Work out the finished part from the listing and answer in its coordinate system (mm). Face numbers are marked on the shaded views. A direction names the side the tool comes from. Coordinates: 2 decimals unless noted, no trailing zeros. Loops run counter-clockwise (first coordinate to the right, second up) from the corner with the lowest first, then second, coordinate; pieces in that order, holes last. Notation, with made-up numbers: M -28.5,-8.5 L 15.5,-8.5 A20 cw 15.5,8.5 Z; hole C -20,40.5 d10. An arc over 180 degrees is marked long. Write each question's results on one line, items separated by ' | '.
```python
from build123d import *

# Parameters (mm, degrees)
SKETCH2_W                    = 57.15
SKETCH2_H                    = 34.925
BASE_FLANGE1_DEPTH           = 3.175
M6_CLEARANCE_HOLE1_D         = 6.6
EDGE_FLANGE2_STRIP_W         = 14.7
EDGE_FLANGE2_STRIP_H         = 3.175
EDGE_FLANGE2_STRIP_CUT_DEPTH = 34.925
EDGE_FLANGE2_DEPTH           = 34.925
CUT_EXTRUDE2_DEPTH           = 79.817416579


# Sheet-metal steps are written as plain solids
with BuildPart() as part:
    # Sketch2 → Base-Flange1 (new body)
    with BuildSketch(Plane.XY):
        Rectangle(SKETCH2_W, SKETCH2_H)
    extrude(amount=BASE_FLANGE1_DEPTH)

    # M6 Clearance Hole1 (through all)
    with Locations(Plane.XY.offset(3.175)):
        with Locations((0, 0)):
            Hole(M6_CLEARANCE_HOLE1_D / 2)

    # Edge-Flange2 strip (across the edge) → Edge-Flange2 strip cut (cut)
    with BuildSketch(Plane(origin=(-28.575, 17.4625, 3.175), x_dir=(1, 0, 0), z_dir=(0, -1, 0))):
        with Locations((-6.35, -1.5875)):
            Rectangle(EDGE_FLANGE2_STRIP_W, EDGE_FLANGE2_STRIP_H)
    extrude(amount=EDGE_FLANGE2_STRIP_CUT_DEPTH, mode=Mode.SUBTRACT)

    # Edge-Flange2 section (across the edge) → Edge-Flange2 (add)
    with BuildSketch(Plane(origin=(-28.575, 17.4625, 3.175), x_dir=(1, 0, 0), z_dir=(0, -1, 0))):
        with BuildLine():
            Line((-3.175, 1), (-3.175, 44.45))
            Line((-3.175, 44.45), (0, 44.45))
            Line((0, 44.45), (0, 1))
            ThreePointArc((0, 1), (0.292893219, 0.292893219), (1, 0))
            Line((1, 0), (1, -3.175))
            ThreePointArc((1, -3.175), (-1.952170811, -1.952170811), (-3.175, 1))
        make_face()
    extrude(amount=EDGE_FLANGE2_DEPTH)

    # Sketch20 → Cut-Extrude2 (cut, through all)
    with BuildSketch(Plane.ZY.offset(31.75)):
        Polygon((4.175, 17.4625), (47.625, -17.4625), (47.625, 17.4625), align=None)
    extrude(amount=-CUT_EXTRUDE2_DEPTH, mode=Mode.SUBTRACT)


solid = part.part
```
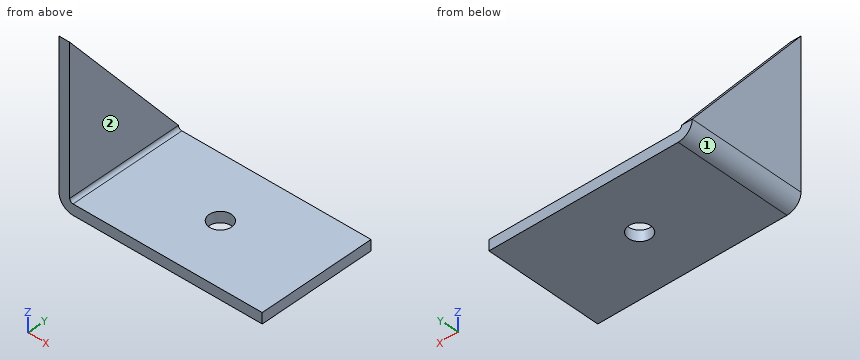
1) Find section D-D, the plane x = -6.5. Give the vertices of the cut face in (y, z) (1 decimal), and give its area (3 significant figures).
Check result:
outline: M -17.5,0 L 17.5,0 L 17.5,3.2 L -17.5,3.2 Z | area: 111 mm^2
2) Which of the six approach directions +Z, -Z, +X, -X, +Y, -Y give full straight-line access (tool end or side, diameter ignored) to the marked faces 1 and 2?
Check result:
face 1: -Z, -X, +Y, -Y | face 2: +Z, +X, +Y, -Y
3) Find section C-C, the plane y = 4. Give the vertices of the cut face in (x, z) (3 decimals).
Check result:
outline: M -31.75,4.175 A4.175 ccw -27.575,0 L 28.575,0 L 28.575,3.175 L -27.575,3.175 A1 cw -28.575,4.175 L -28.575,20.924 L -31.75,20.924 Z
4) Given pin 1 Ø12 at (x, y) = (-1.5, -10) entering from +Z (3 decimals); pin 2 Ø5 at (y, z) = (-0.5, 20.5) entering from +X (3 decimals), each flat-ended and moving along its own axis, determine where each tip first touches the part or whether it passes through.
Check result:
pin 1: z = 3.175 | pin 2: x = -28.575
5) Straight lines are drawn through the part: probe 1 along Y at (x, z) = (0, 1.4); probe 2 along Z at (x, y) = (3.5, 14.5) (3 decimals); probe 3 along X at (y, z) = (-3, 28) (3 decimals). For each, find the intervals that lie inside material, in ascending order. Write a range as [from, to].
Check result:
probe 1: [-17.46, -3.3], [3.3, 17.46] | probe 2: [0, 3.175] | probe 3: [-31.75, -28.575]
6) Find section A-A, the plane y = 0. Give the vertices of the cut face in (x, z) (3 decimals), and give its area (3 significant figures).
Check result:
outline: M -31.75,4.175 A4.175 ccw -27.575,0 L -3.3,0 L -3.3,3.175 L -27.575,3.175 A1 cw -28.575,4.175 L -28.575,25.9 L -31.75,25.9 Z; M 3.3,0 L 28.575,0 L 28.575,3.175 L 3.3,3.175 Z | area: 239 mm^2
7) Find section B-B, the plane x = 0. Give the vertices of the cut face in (y, z) (1 decimal), and give its area (3 significant figures).
Check result:
outline: M -17.5,0 L -3.3,0 L -3.3,3.2 L -17.5,3.2 Z; M 3.3,0 L 17.5,0 L 17.5,3.2 L 3.3,3.2 Z | area: 89.9 mm^2
